Answer from the drawing. Dimensions are ordinates in mm from the lowest x, y and z of the part. Coordinates: 2 decimals unless noted, no trailing zeros. Loops run counter-clockwise (first coordinate to the right, second up) from the corner with the lowest first, then second, coordinate; pieces in that order, holes last.
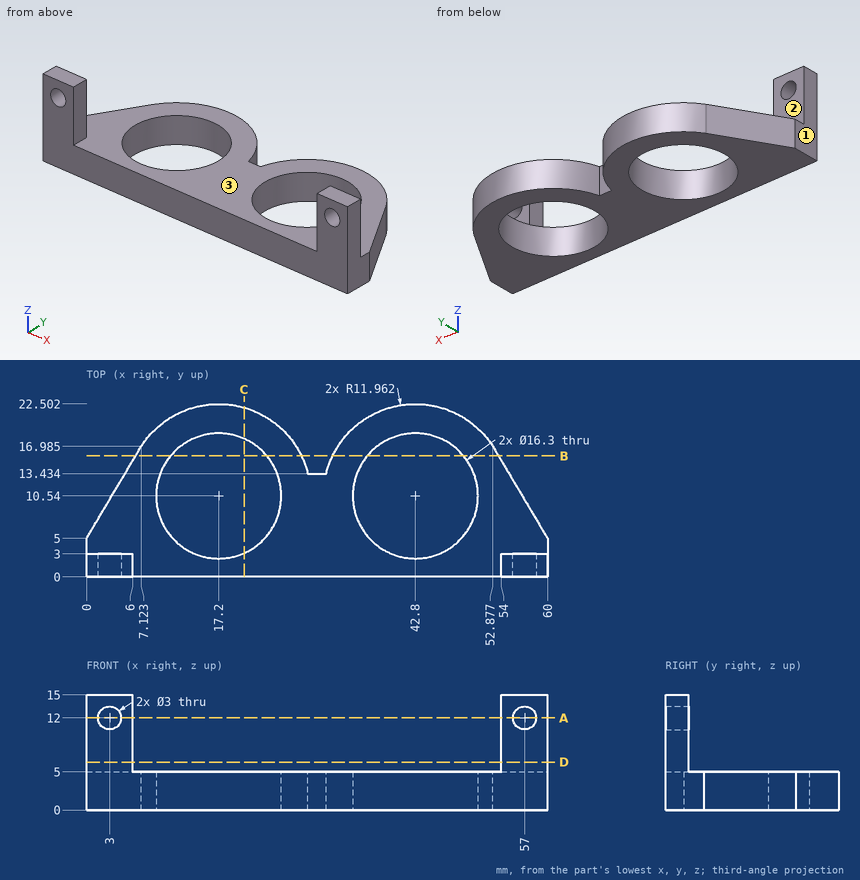
Item 1: Determine the mould class of the marked faces 1, 2 and 3 for opening direction X: released by +X, released by -X, zero draft, split by the parting line, or undercut.
Numbers:
face 1: released by -X
face 2: zero draft
face 3: undercut
Item 2: A cutting plane is placed at C-C on x = 20.5. Determine the outline of the cut face in (y, z).
Numbers:
outline: (0, 0) - (3.09, 0) - (3.09, 5) - (0, 5) - close; (17.99, 0) - (22.04, 0) - (22.04, 5) - (17.99, 5) - close
Item 3: A cutting plane is placed at D-D on z = 6.25. Determine the outline of the cut face in (x, y), then the cut area to 3 significant figures.
Numbers:
outline: (0, 0) - (6, 0) - (6, 3) - (0, 3) - close; (54, 0) - (60, 0) - (60, 3) - (54, 3) - close
area: 36.0 mm2
Item 4: Find the intervals of material crossed by line 1 along X through (y, z) = (1.35, 12); line 2 along X through (y, z) = (11.5, 1.5); line 3 along X through (y, z) = (3.75, 4), in increasing order.
Numbers:
line 1: x = 0 to 1.5, 4.5 to 6, 54 to 55.5, 58.5 to 60
line 2: x = 3.86 to 9.11, 25.29 to 34.71, 50.89 to 56.14
line 3: x = 0 to 12.69, 21.71 to 38.29, 47.31 to 60
Item 5: A cutting plane is placed at B-B on y = 15.75. Determine the outline of the cut face in (x, z).
Numbers:
outline: (6.39, 0) - (10.93, 0) - (10.93, 5) - (6.39, 5) - close; (23.47, 0) - (27.97, 0) - (27.97, 5) - (23.47, 5) - close; (32.03, 0) - (36.53, 0) - (36.53, 5) - (32.03, 5) - close; (49.07, 0) - (53.61, 0) - (53.61, 5) - (49.07, 5) - close
Item 6: Given pin 1 (8 mm diameter, centred on x = 36.5, z = 2.5, fed in from +Y); pin 2 (3 mm diameter, centred on x = 4.5, z = 12, fed in from +Y); pin 3 (3 mm diameter, centred on x = 8, y = 16.5, fed in from +Z); pin 4 (10 mm diameter, centred on x = 42.8, y = 10.54, fed in from -Z), each flat-ended and moving along its own axis, determine where each tip first touches the part or whether it passes through.
Numbers:
pin 1: stops at y = 22.28
pin 2: stops at y = 3
pin 3: stops at z = 5
pin 4: passes through
Item 7: A cutting plane is placed at A-A on z = 12. Determine the outline of the cut face in (x, y), then the cut area to 3 significant figures.
Numbers:
outline: (0, 0) - (1.5, 0) - (1.5, 3) - (0, 3) - close; (4.5, 0) - (6, 0) - (6, 3) - (4.5, 3) - close; (54, 0) - (55.5, 0) - (55.5, 3) - (54, 3) - close; (58.5, 0) - (60, 0) - (60, 3) - (58.5, 3) - close
area: 18.0 mm2
